Part model, mm, in its own coordinate system. Face numbers are marked on the shaded views. A direction names the side the tool comes from. Round coordinates to 2 decimals unless told otherwise and drop trailing zeros. Loops run counter-clockwise (first coordinate to the right, second up) from the corner with the lowest first, then second, coordinate; pieces in that order, holes last. Notation, with made-up numbers: M 66,60 L 95,60 A17 ccw 95,66 Z; hole C -7,-26 d9. An arc over 180 degrees is marked long. Answer as CSV lines item,"result". Start each with the question number.
Item 1: Wall check: line 1 (Z direction, x = 50, y = -13.5); line 2 (Z direction, x = 11, y = -15.5); line 3 (Y direction, x = 1, z = 19). Give the ranges that are in metal, low to high.
Item 2: Band-saw the part on C-C (x = 56). Give the cut face in (y, z), and give its area (3 significant figures).
Item 3: Drop flat-ended pins along their axis: pin 1 Ø5 at (x, y) = (51, 16.5) entering from -Z; pin 2 Ø19 at (x, y) = (28, 2.5) entering from +Z; pin 3 Ø1.5 at (y, z) = (20.5, 15) entering from +X. Give the stop position or say it passes through.
Item 4: Band-saw the part on B-B (z = 19.5). Give the cut face in (x, y).
Item 5: Band-saw the part on A-A (y = -1). Give the cut face in (x, z).
Item 6: Band-saw the part on D-D (y = -22.5). Give the cut face in (x, z), and give its area (3 significant figures).
Item 7: Which spindle directions (+Z, -Z, +X, -X, +Y, -Y) get a long thin tool onto all of the face, cutting with end or side? Do the marked faces 1, 2 and 3. Say none if no direction does.
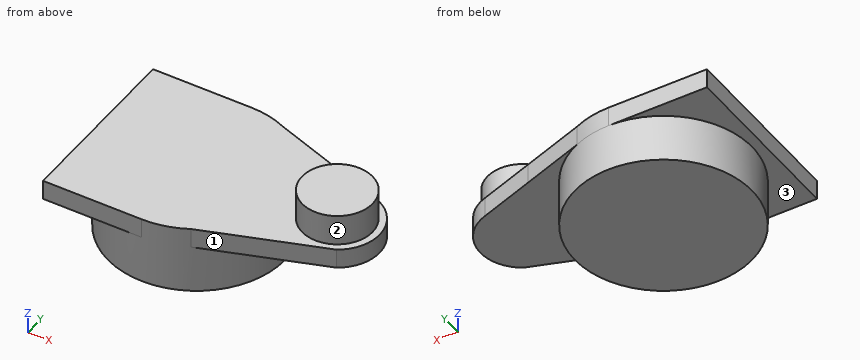
```python
from build123d import *

# Parameters (mm, degrees)
SKETCH1_R           = 31.5
BOSS_EXTRUDE1_DEPTH = 17
SKETCH2_R           = 31.5
BOSS_EXTRUDE2_DEPTH = 7
SKETCH3_R           = 12.5
BOSS_EXTRUDE3_DEPTH = 11


with BuildPart() as part:
    # Sketch1 → Boss-Extrude1 (new body)
    with BuildSketch(Plane.XY):
        Circle(SKETCH1_R)
    extrude(amount=BOSS_EXTRUDE1_DEPTH)

    # Sketch2 → Boss-Extrude2 (add)
    with BuildSketch(Plane.XY.offset(17)):
        with BuildLine():
            Line((0, 31.5), (-35, 31.5))
            Line((-35, 31.5), (-35, -31.5))
            Line((-35, -31.5), (0, -31.5))
            ThreePointArc((0, -31.5), (-31.5, 0), (0, 31.5))
        make_face()
        with Locations(Location((0, 0, 0), (0, 0, 90))):
            Circle(SKETCH2_R)
        with BuildLine():
            Line((35, 21.078091868), (12.801393416, 28.78149278))
            ThreePointArc((12.801393416, 28.78149278), (26.414900081, 17.161091274), (31.5, 0))
            ThreePointArc((31.5, 0), (27.098152806, -16.060514142), (15.122849874, -27.632397864))
            Line((15.122849874, -27.632397864), (57.643936691, -12.906209043))
            ThreePointArc((57.643936691, -12.906209043), (64.905048238, 1.685092584), (54.569602713, 14.28701267))
            Line((54.569602713, 14.28701267), (35, 21.078091868))
        make_face()
    extrude(amount=BOSS_EXTRUDE2_DEPTH)

    # Sketch3 → Boss-Extrude3 (add)
    with BuildSketch(Plane.XY.offset(24)):
        with Locations((50, 0)):
            Circle(SKETCH3_R)
    extrude(amount=BOSS_EXTRUDE3_DEPTH)


solid = part.part
```
Answer block:
1,line 1,"z = 17 to 24"
1,line 2,"z = 0 to 24"
1,line 3,"y = -31.48 to 31.48"
2,outline,"M -13.48,17 L 13.75,17 L 13.75,24 L 10.97,24 L 10.97,35 L -10.97,35 L -10.97,24 L -13.48,24 Z"
2,area,"432 mm^2"
3,pin 1,"stops at z = 17"
3,pin 2,"stops at z = 24"
3,pin 3,"stops at x = 24.54"
4,outline,"M -35,-31.5 L 0,-31.5 A31.5 ccw 15.12,-27.63 L 57.64,-12.91 A15 ccw 54.57,14.29 L 12.8,28.78 A31.5 ccw 0,31.5 L -35,31.5 Z"
5,outline,"M -35,17 L -31.48,17 L -31.48,0 L 31.48,0 L 31.48,17 L 64.97,17 L 64.97,24 L 62.46,24 L 62.46,35 L 37.54,35 L 37.54,24 L -35,24 Z"
6,outline,"M -35,17 L -22.05,17 L -22.05,0 L 22.05,0 L 22.05,17 L 29.94,17 L 29.94,24 L -35,24 Z"
6,area,"1,200 mm^2"
7,face 1,"+Z, -Z, +X, -Y"
7,face 2,"+Z"
7,face 3,"-Z, -X"
